from build123d import *

# Parameters (mm, degrees)
SKETCH075_R           = 23
PAD030_DEPTH          = 2
SKETCH076_W           = 3
SKETCH076_H           = 2
POCKET040_DEPTH       = 5
POLARPATTERN004_COUNT = 5


with BuildPart() as part:
    # Sketch075 → Pad030 (new body)
    with BuildSketch(Plane.XY):
        Circle(SKETCH075_R)
    extrude(amount=PAD030_DEPTH)

    # Sketch076 → Pocket040 (cut)
    with BuildSketch(Plane(origin=(0, -18, 0), x_dir=(0, 1, 0), z_dir=(0, 0, 1))):
        with Locations((0, 3.5)):
            Rectangle(SKETCH076_W, SKETCH076_H)
        with Locations((0, -3.5)):
            Rectangle(SKETCH076_W, SKETCH076_H)
    pocket040 = extrude(amount=POCKET040_DEPTH, mode=Mode.SUBTRACT)

    # PolarPattern004: Pocket040 ×5 about axis
    polarpattern004_axis = Axis((0, 0, 0), (0, 0, 1))
    for i in range(1, POLARPATTERN004_COUNT):
        add(pocket040.rotate(polarpattern004_axis, i * 360 / POLARPATTERN004_COUNT), mode=Mode.SUBTRACT)


solid = part.part
CAD build for the part. Positions are in the model's coordinates, mm. Round coordinates to 2 decimals unless told otherwise and drop trailing zeros. Write each loop counter-clockwise with the first axis right and the second up, starting at its lowest first coordinate (ties: lowest second). Pieces come first, ordered by that corner, then holes. Notation, with made-up numbers: M 67,28.5 L 116,28.5 A16 cw 116,44.5 Z; hole C -31.5,46 d1. An arc over 180 degrees is marked long. Use a Markdown table: item, result. Add a question column.
1. Drill centre lines: probe 1 along X at (y, z) = (-18, 0.8); probe 2 along X at (y, z) = (17.5, 0.5); probe 3 along Y at (x, z) = (19, 1.35). Where is each one in solid material? Low to high.
2. Slice it at C-C on y = 7. Give the cut face in (x, z).
3. Slice it at B-B on z = 1.65. Give the number of separate pieces and of enclosed holes in the cut face, then the cut area to 3 significant figures.
4. Slice it at A-A on y = 12.5. Give the cut face in (x, z), then the cut area to 3 significant figures.
5. Slice it at D-D on y = 20. Give the cut face in (x, z).
6. Flat gauge pins, fed straight in: P1, Ø1, axis at x = 3, z = 0.5, coming from the +Y side; P2, Ø1, axis at y = -17.5, z = 1, coming from the +X side; P3, Ø1, axis at y = -17.5, z = 1, coming from the -X side; P4, Ø8, axis at x = 0, y = -16.5, coming from the -Z side. Where does each tip first touch, or does it go through?
7. Pull direction Y, two halves, no side cores. Call faces 1 (the face through (0, 0, 2)), 2 (the face through (-16.366, -7.946, 0.986)): released by +Y, released by -Y, zero draft, split by the parting line, or undercut.
Reply:
| question | item | result |
|---|---|---|
| 1 | probe 1 | x = -14.32 to -4.5, -2.5 to 2.5, 4.5 to 14.32 |
| 1 | probe 2 | x = -14.92 to -9.09, -7.15 to 7.15, 9.09 to 14.92 |
| 1 | probe 3 | y = -12.96 to -3.54, -1.44 to 12.96 |
| 2 | outline | M -21.91,0 L 21.91,0 L 21.91,2 L -21.91,2 Z |
| 3 | separate pieces | 1 |
| 3 | enclosed holes | 10 |
| 3 | area | 1,600 mm^2 |
| 4 | outline | M -19.31,0 L -14.64,0 L -14.64,2 L -19.31,2 Z; M -12.17,0 L 12.17,0 L 12.17,2 L -12.17,2 Z; M 14.64,0 L 19.31,0 L 19.31,2 L 14.64,2 Z |
| 4 | area | 67.3 mm^2 |
| 5 | outline | M -11.36,0 L 11.36,0 L 11.36,2 L -11.36,2 Z |
| 6 | P1 | stops at y = 22.86 |
| 6 | P2 | stops at x = 15.49 |
| 6 | P3 | stops at x = -15.49 |
| 6 | P4 | stops at z = 0 |
| 7 | face 1 | zero draft |
| 7 | face 2 | undercut |
